Could you check a few things on this model? Use its own coordinates, in mm. Face numbers are marked on the shaded views. Coordinates: 2 decimals unless noted, no trailing zeros. Loops run counter-clockwise (first coordinate to the right, second up) from the corner with the lowest first, then second, coordinate; pieces in that order, holes last. Notation, with made-up numbers: (-30, 60) -> (9, 60) arc R24 ccw to (9, 91) -> close; hole circle Ø10 at (38, 68.25). An arc over 180 degrees is marked (long way). One line per question, with ' | ' between items.
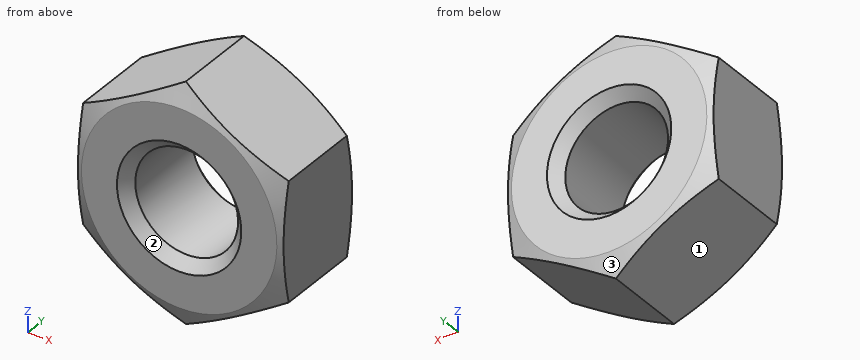
from build123d import *

# Parameters (mm, degrees)
BOSS_EXTRUDE1_DEPTH = 2.5


with BuildPart() as part:
    # Sketch1 → Boss-Extrude1 (new, symmetric)
    with BuildSketch(Plane(origin=(0, 0, 0), x_dir=(1, 0, 0), z_dir=(0, 1, 0))):
        Polygon((0, 5.773502692), (-5, 2.886751346), (-5, -2.886751346), (0, -5.773502692), (5, -2.886751346), (5, 2.886751346), align=None)
    extrude(amount=BOSS_EXTRUDE1_DEPTH, both=True)

    # Sketch2 → Cut-Revolve1 (revolve, cut)
    with BuildSketch(Plane.XY, mode=Mode.PRIVATE) as cut_revolve1_sk:
        Polygon((-4.75274654, 2.5), (-5.825, 2), (-5.825, 2.5), align=None)
    cut_revolve1 = revolve(cut_revolve1_sk.sketch.rotate(Axis((0, 0, 0), (0, 1, 0)), 270), axis=Axis((0, 0, 0), (0, 1, 0)), mode=Mode.SUBTRACT)

    # Mirror1: Cut-Revolve1 across plane
    add(cut_revolve1.mirror(Plane.ZX), mode=Mode.SUBTRACT)

    # Sketch4 → M6 Tapped Hole1 (revolve, cut)
    with BuildSketch(Plane(origin=(0, 2.5, 0), x_dir=(0, 0, 1), z_dir=(1, 0, 0))):
        Polygon((0, 0), (0, 5), (3.025, 5), (2.5, 4.475), (2.5, 0.525), (3.025, 0), align=None)
    revolve(axis=Axis((0, 8.85, 0), (0, -1, 0)), mode=Mode.SUBTRACT)


solid = part.part
1) We'd pull the mould along Z, two halves only. Please class the marked faces 1, 2 and 3: pulls with the +Z half, pulls with the -Z half, needs draft (parallel to the pull), parting line crosses it, or undercut.
Data:
face 1: pulls with the -Z half | face 2: undercut | face 3: parting line crosses it
2) If we section it at B-B on y = 1.65: Please give me the cut outline in (x, z), and give its area (3 significant figures).
Data:
outline: (-5, -2.89) -> (0, -5.77) -> (5, -2.89) -> (5, 2.89) -> (0, 5.77) -> (-5, 2.89) -> close; hole circle Ø5 at (0, 0) | area: 67.0 mm²
3) I need wall thicknesses on line 1 along X through (y, z) = (0.9, 0); line 2 along Z through (x, y) = (0.75, 0.7); line 3 along Z through (x, y) = (-2.25, 1.55). Which ranges of each line are inside material? Lowest first, please. Write a range as from..to.
Data:
line 1: -5..-2.5, 2.5..5 | line 2: -5.34..-2.38, 2.38..5.34 | line 3: -4.47..-1.09, 1.09..4.47
4) I'm going to push flat-ended pins straight in: pin 1 Ø1 at (x, z) = (-2, 0.5) entering from +Y; pin 2 Ø1.5 at (y, z) = (-0.5, 4) entering from -X. Where does each tip first touch, or does it pass through?
Data:
pin 1: y = 2.04 | pin 2: x = -4.37
5) If we section it at A-A on z = 0: Please give me the cut outline in (x, y) (3 decimals).
Data:
outline: (-5, -2.385) -> (-4.753, -2.5) -> (-3.025, -2.5) -> (-2.5, -1.975) -> (-2.5, 1.975) -> (-3.025, 2.5) -> (-4.753, 2.5) -> (-5, 2.385) -> close; (2.5, -1.975) -> (3.025, -2.5) -> (4.753, -2.5) -> (5, -2.385) -> (5, 2.385) -> (4.753, 2.5) -> (3.025, 2.5) -> (2.5, 1.975) -> close
